Can you work these out from the model? Positions are in its coordinate system, mm. Face numbers are marked on the shaded views. A direction names the side the tool comes from. Give positions to 0.01 mm unless a question says otherwise; leave off trailing zeros. Loops run counter-clockwise (first coordinate to the right, second up) from the corner with the lowest first, then second, coordinate; pieces in that order, holes last. Notation, with made-up numbers: M 11.5,44.5 L 33.5,44.5 A28 cw 33.5,63.5 Z; hole C 32.25,-36.5 d2. An arc over 180 degrees is marked long. Put each result on its own line as item: value. Start each with the question number.
1) For the marked faces 1 and 2, which set-ups out of +Z, -Z, +X, -X, +Y, -Y let a thin tool reach every point of the face, with its end or its side?
2) Please list where this line runs through material, in increasing order: line 1 along Y through (x, z) = (60.5, 1). Write a range as from..to.
3) Imagine slicing it at C-C (y = 9). Write out the boundary of the cut face in (x, z), then the cut area to 3 significant figures.
4) Imagine slicing it at B-B (z = 7.5). Write out the boundary of the cut face in (x, y).
5) For P1, Ø7.5, axis at x = 36, z = 5, coming from the +Y side; P2, Ø4, axis at y = 31, z = 12.5, coming from the +X side, each with a flat end and sliding along its axis, tell me the tip position at first contact or that it passes through.
6) Imagine slicing it at A-A (x = 20). Write out the boundary of the cut face in (y, z), then the cut area to 3 significant figures.
from build123d import *

# Parameters (mm, degrees)
F1_DEPTH = 15
F4_DEPTH = 3.201
F5_DEPTH = 3.201
F6_R     = 2


with BuildPart() as f1:
    # F0 (on Top) → F1 (new body)
    with BuildSketch(Plane.XY):
        Polygon((3.2, 35), (0, 35), (0, 0), (70, 0), (70, 3.2), (3.2, 3.2), align=None)
    extrude(amount=F1_DEPTH)

    # F2 (on face) → F4 (cut, through all)
    with BuildSketch(Plane(origin=(0, 3.2, 0), x_dir=(-1, 0, 0), z_dir=(0, 1, 0))):
        with BuildLine():
            Line((-15.2, 10.75), (-28.7, 10.75))
            ThreePointArc((-28.7, 10.75), (-31.95, 7.5), (-28.7, 4.25))
            Line((-28.7, 4.25), (-15.2, 4.25))
            ThreePointArc((-15.2, 4.25), (-11.95, 7.5), (-15.2, 10.75))
        make_face()
        with BuildLine():
            Line((-58.2, 4.25), (-44.7, 4.25))
            ThreePointArc((-44.7, 4.25), (-41.45, 7.5), (-44.7, 10.75))
            Line((-44.7, 10.75), (-58.2, 10.75))
            ThreePointArc((-58.2, 10.75), (-61.45, 7.5), (-58.2, 4.25))
        make_face()
    extrude(amount=-F4_DEPTH, mode=Mode.SUBTRACT)

    # F3 (on face) → F5 (cut, through all)
    with BuildSketch(Plane.YZ.offset(3.2)):
        with BuildLine():
            Line((23.7, 10.75), (15.2, 10.75))
            ThreePointArc((15.2, 10.75), (11.95, 7.5), (15.2, 4.25))
            Line((15.2, 4.25), (23.7, 4.25))
            ThreePointArc((23.7, 4.25), (26.95, 7.5), (23.7, 10.75))
        make_face()
    extrude(amount=-F5_DEPTH, mode=Mode.SUBTRACT)

    # F6
    f6_edges = [f1.edges().sort_by_distance(p)[0] for p in [
        (70, 1.6, 15),
        (70, 1.6, 0),
        (1.6, 35, 15),
        (1.6, 35, 0),
    ]]
    fillet(f6_edges, radius=F6_R)


solid = f1.part
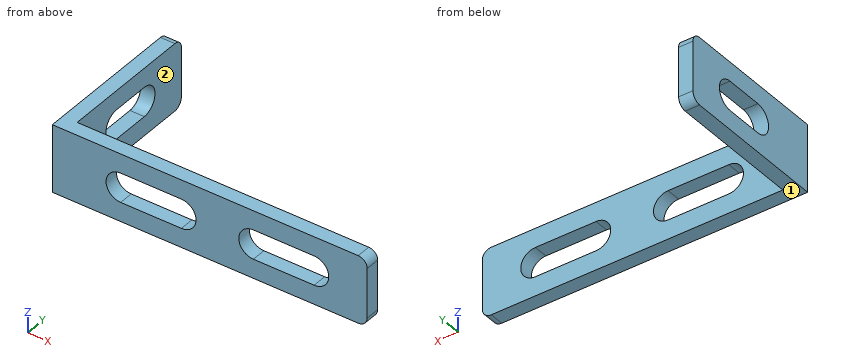
Recorded:
1. face 1: -Z, +X, -X, +Y, -Y
1. face 2: +Z, -Z, +X, +Y
2. line 1: 0..3.2
3. outline: M 0,0 L 3.2,0 L 3.2,15 L 0,15 Z
3. area: 48.0 mm²
4. outline: M 0,0 L 11.95,0 L 11.95,3.2 L 3.2,3.2 L 3.2,11.95 L 0,11.95 Z; M 0,26.95 L 3.2,26.95 L 3.2,35 L 0,35 Z; M 31.95,0 L 41.45,0 L 41.45,3.2 L 31.95,3.2 Z; M 61.45,0 L 70,0 L 70,3.2 L 61.45,3.2 Z
5. P1: y = 3.2
5. P2: x = 3.2
6. outline: M 0,0 L 3.2,0 L 3.2,4.25 L 0,4.25 Z; M 0,10.75 L 3.2,10.75 L 3.2,15 L 0,15 Z
6. area: 27.2 mm²
